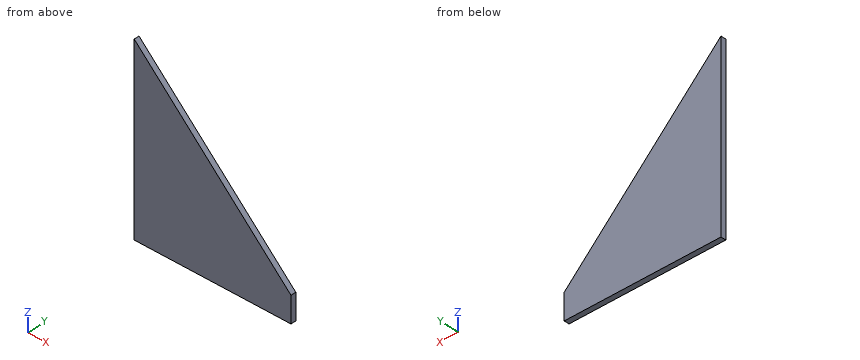
from build123d import *

# Parameters (mm, degrees)
F0_W     = 152.4
F0_H     = 152.4
F1_DEPTH = 5.08
F3_DEPTH = 5.08
F4_DEPTH = 25.4


with BuildPart() as f1:
    # F0 (on Front) → F1 (new body)
    with BuildSketch(Plane.XZ):
        with Locations((-93.7180127949, 26.5866962026)):
            Rectangle(F0_W, F0_H)
    extrude(amount=F1_DEPTH)

    # F2 (on face) → F3 (cut)
    with BuildSketch(Plane.XZ.offset(5.08)):
        Polygon((-17.5180127949, 102.7866962026), (-169.9180127949, 102.7866962026), (-17.5180127949, -49.6133037974), align=None)
    extrude(amount=-F3_DEPTH, mode=Mode.SUBTRACT)

    # F4 (add): a face of the model
    f4_faces = [f1.faces().sort_by_distance(p)[0] for p in [
        (-93.7180127949, -2.54, -49.6133037974),
    ]]
    extrude(f4_faces, amount=F4_DEPTH)


solid = f1.part
Can you work these out from the model? Positions are in its coordinate system, mm. Coordinates: 2 decimals unless noted, no trailing zeros. Write each loop counter-clockwise with the first axis right and the second up, starting at its lowest first coordinate (ties: lowest second). Pieces come first, ordered by that corner, then holes. Notation, with made-up numbers: (-24, -39) -> (8, -39) arc R9 cw to (8, -31) -> close; hole circle Ø2 at (72, 28). An arc over 180 degrees is marked (long way). Answer as CSV lines item,"result".
1) Will this pin go through, and if not, where does the flat tip stop? P1, Ø3, axis at x = -115, y = -2, coming from the +Z side.
Check result:
P1,"z = 49.37"
2) If we section it at A-A on y = -2.7: Please give me the cut outline in (x, z).
Check result:
outline,"(-169.92, -75.01) -> (-17.52, -75.01) -> (-17.52, -49.61) -> (-169.92, 102.79) -> close"
3) If we section it at B-B on x = -33: Please give me the cut outline in (y, z).
Check result:
outline,"(-5.08, -75.01) -> (0, -75.01) -> (0, -34.13) -> (-5.08, -34.13) -> close"
4) If I drill on line 1 (Z direction, x = -99.5, y = -0.95); line 2 (Z direction, x = -90, y = -4.4); line 3 (X direction, y = -0.15, z = 19.5), over which ranges is the centre line in solid material (lowest first)? Write a range as from..to.
Check result:
line 1,"-75.01..32.37"
line 2,"-75.01..22.87"
line 3,"-169.92..-86.63"
